Check sheet for the drawn part. Datum: minimum x, y, z corner. Units: mm. A direction names the side the tool comes from. Coordinates: 2 decimals unless noted, no trailing zeros. Order: outer loops, then holes, each group sorted by start corner. A loop starts at its lowest first (then second) coordinate and runs counter-clockwise, first axis right, second up. Notation, with made-up numbers: (89, 49.25) - (140, 49.25) arc R21 ccw to (140, 82.25) - close; hole circle Ø11 at (-8.5, 57). An arc over 180 degrees is marked (long way). Return JSON: item names as keys, results as strings. Group by question number.
Item 1: Section check C-C on z = 14. Enter the section's corners in (x, y).
Item 2: Section check A-A on y = 18. Enter the section's corners in (x, z).
Item 3: Section check D-D on z = 55. Enter the section's corners in (x, y), then the cut area to 3 significant figures.
Item 4: Gauge pin test, flat ends, axial feed: pin 1 (5 mm diameter, centred on x = 18, y = 18, fed in from +Z); pin 2 (10 mm diameter, centred on x = 27, y = 6, fed in from -Z); pin 3 (6 mm diameter, centred on y = 24, z = 34.5, fed in from -X); pin 4 (4 mm diameter, centred on x = 24.5, z = 29.5, fed in from -Y). Record the tip position at first contact, or that the pin passes through.
Item 5: Scan lines: probe 1 along Y at (x, z) = (18, 13); probe 2 along Y at (x, z) = (18, 45); probe 3 along Z at (x, y) = (33, 24). Record each from-to range of solid material in increasing order.
Item 6: Tool access check on the marked faces 1 and 2. Record the directions out of +Z, -Z, +X, -X, +Y, -Y that give a thin tool (end or side, any length) a straight path to the whole face; none if there is none.
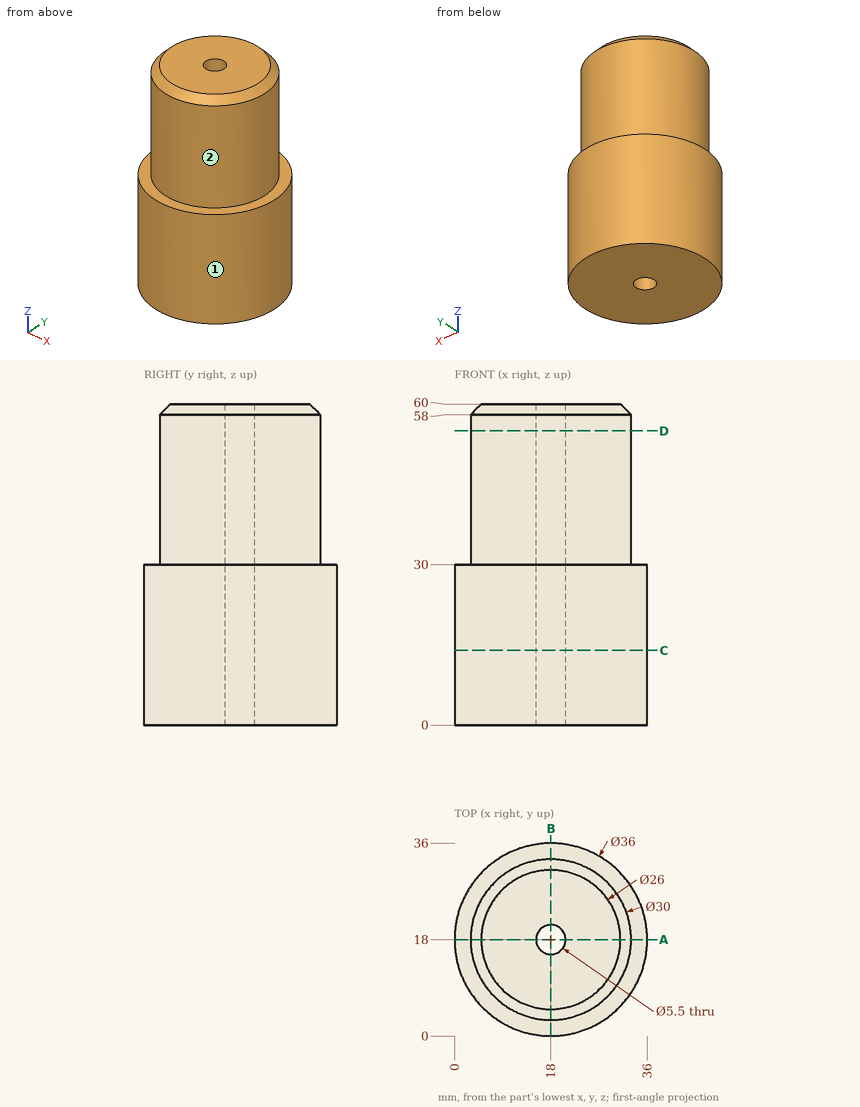
Computed:
{
 "1": {"outline": "circle Ø36 at (18, 18); hole circle Ø5.5 at (18, 18)"},
 "2": {"outline": "(0, 0) - (15.25, 0) - (15.25, 60) - (5, 60) - (3, 58) - (3, 30) - (0, 30) - close; (20.75, 0) - (36, 0) - (36, 30) - (33, 30) - (33, 58) - (31, 60) - (20.75, 60) - close"},
 "3": {"outline": "circle Ø30 at (18, 18); hole circle Ø5.5 at (18, 18)", "area": "683 mm²"},
 "4": {"pin 1": "passes through", "pin 2": "stops at z = 0", "pin 3": "stops at x = 3.3", "pin 4": "stops at y = 0.57"},
 "5": {"probe 1": "y = 0 to 15.25, 20.75 to 36", "probe 2": "y = 3 to 15.25, 20.75 to 33", "probe 3": "z = 0 to 30"},
 "6": {"face 1": "+Z, -Z", "face 2": "+Z"}
}
